Autodesk Inventor part; units mm, degrees
ref_plane "Work Plane1" through (12.7, 0, 0) normal (1, 0, 0) x (0, 1, 0)
ref_plane "Work Plane2" through (0, 12.7, 0) normal (0, 1, 0) x (-1, 0, 0)
ref_plane "Work Plane3" through (0, 0, -12.7) normal (0, 0, 1) x (1, 0, 0)
sketch "Sketch1" plane through (0, 0, 0) normal (0, 1, 0) x (-1, 0, 0)
  line L0 (0, 0) -> (-25.4, 0)
  line L1 (-25.4, 0) -> (-25.4, -25.4)
  line L2 (-25.4, -25.4) -> (0, -25.4)
  line L3 (0, -25.4) -> (0, 0)
  dimension "d0" = 25.4
  dimension "d1" = 25.4
extrude "Extrusion1" add sketch "Sketch1" along normal blind 25.4
sketch "Sketch3" plane through (25.4, 0, 0) normal (1, 0, 0) x (0, 0, -1)
  line L0 (0, 25.4) -> (8.4582, 25.4)
  line L1 (8.4582, 25.4) -> (8.4582, 16.9418)
  line L2 (8.4582, 16.9418) -> (0, 16.9418)
  line L3 (0, 16.9418) -> (0, 25.4)
  line L4 (0, 0) -> (8.4582, 0)
  line L5 (8.4582, 0) -> (8.4582, 8.4582)
  line L6 (8.4582, 8.4582) -> (0, 8.4582)
  line L7 (0, 8.4582) -> (0, 0)
  line L8 (0, 0) -> (25.4, 0)
  line L9 (25.4, 0) -> (16.9418, 0)
  line L10 (16.9418, 0) -> (16.9418, 8.4582)
  line L11 (16.9418, 8.4582) -> (25.4, 8.4582)
  line L12 (25.4, 8.4582) -> (25.4, 0)
  line L13 (0, 25.4) -> (25.4, 25.4)
  line L14 (25.4, 25.4) -> (16.9418, 25.4)
  line L15 (16.9418, 25.4) -> (16.9418, 16.9418)
  line L16 (16.9418, 16.9418) -> (25.4, 16.9418)
  line L17 (25.4, 16.9418) -> (25.4, 25.4)
  line L18 (8.4582, 25.4) -> (16.9418, 25.4)
  line L19 (16.9418, 25.4) -> (16.9418, 0)
  line L20 (16.9418, 0) -> (8.4582, 0)
  line L21 (8.4582, 0) -> (8.4582, 25.4)
  line L22 (0, 16.9418) -> (25.4, 16.9418)
  line L23 (25.4, 16.9418) -> (25.4, 8.4582)
  line L24 (25.4, 8.4582) -> (0, 8.4582)
  line L25 (0, 8.4582) -> (0, 16.9418)
  dimension "d4" = 8.4582
  dimension "d5" = 8.4582
  dimension "d6" = 8.4582
  dimension "d7" = 8.4582
  dimension "d8" = 8.4582
  dimension "d9" = 8.4582
  dimension "d10" = 8.4582
  dimension "d11" = 8.4582
extrude "Extrusion2" cut sketch "Sketch3" against normal blind 2.54 contours L13 L15 L22 L1 | L2 L21 L6 L25 | L22 L19 L24 L21 | L24 L10 L8 L5 | L16 L23 L11 L19
sketch "Sketch5" plane through (25.4, 0, -25.4) normal (0, 0, -1) x (-1, 0, 0)
  line L0 (25.4, 0) -> (25.4, 25.4)
  line L1 (25.4, 0) -> (16.9418, 0)
  line L2 (16.9418, 0) -> (16.9418, 8.4582)
  line L3 (16.9418, 8.4582) -> (25.4, 8.4582)
  line L4 (25.4, 8.4582) -> (25.4, 0)
  line L5 (0, 0) -> (8.4582, 0)
  line L6 (8.4582, 0) -> (8.4582, 8.4582)
  line L7 (8.4582, 8.4582) -> (0, 8.4582)
  line L8 (0, 8.4582) -> (0, 0)
  line L9 (2.54, 25.4) -> (0, 25.4)
  line L10 (0, 25.4) -> (8.4582, 25.4)
  line L11 (8.4582, 25.4) -> (8.4582, 16.9418)
  line L12 (8.4582, 16.9418) -> (0, 16.9418)
  line L13 (0, 16.9418) -> (0, 25.4)
  line L14 (0, 25.4) -> (25.4, 25.4)
  line L15 (25.4, 25.4) -> (16.9418, 25.4)
  line L16 (16.9418, 25.4) -> (16.9418, 16.9418)
  line L17 (16.9418, 16.9418) -> (25.4, 16.9418)
  line L18 (25.4, 16.9418) -> (25.4, 25.4)
  line L19 (0, 8.4582) -> (2.54, 8.4582)
  line L20 (0, 8.4582) -> (25.4, 8.4582)
  line L21 (25.4, 8.4582) -> (25.4, 16.9418)
  line L22 (25.4, 16.9418) -> (0, 16.9418)
  line L23 (0, 16.9418) -> (0, 8.4582)
  line L24 (8.4582, 25.4) -> (16.9418, 25.4)
  line L25 (16.9418, 25.4) -> (16.9418, 0)
  line L26 (16.9418, 0) -> (8.4582, 0)
  line L27 (8.4582, 0) -> (8.4582, 25.4)
  dimension "d14" = 8.4582
  dimension "d15" = 8.4582
  dimension "d16" = 8.4582
  dimension "d17" = 8.4582
  dimension "d18" = 8.4582
  dimension "d19" = 8.4582
  dimension "d20" = 8.4582
  dimension "d21" = 8.4582
extrude "Extrusion3" cut sketch "Sketch5" against normal blind 2.54 contours L3 L25 L17 L0 | L26 L6 L20 L2 | L20 L27 L22 L25 | L22 L11 L14 L16 | L7 L23 L12 L27
sketch "Sketch7" plane through (0, 0, 0) normal (0, -1, 0) x (1, 0, 0)
  line L0 (25.4, -16.9418) -> (25.4, -25.4)
  line L1 (25.4, -25.4) -> (16.9418, -25.4)
  line L2 (16.9418, -25.4) -> (16.9418, -16.9418)
  line L3 (16.9418, -16.9418) -> (25.4, -16.9418)
  line L4 (25.4, -16.9418) -> (25.4, -25.4)
  line L5 (8.4582, -25.4) -> (0, -25.4)
  line L6 (0, -25.4) -> (8.4582, -25.4)
  line L7 (8.4582, -25.4) -> (8.4582, -16.9418)
  line L8 (8.4582, -16.9418) -> (0, -16.9418)
  line L9 (0, -16.9418) -> (0, -25.4)
  line L10 (25.4, -8.4582) -> (25.4, 0)
  line L11 (25.4, 0) -> (16.9418, 0)
  line L12 (16.9418, 0) -> (16.9418, -8.4582)
  line L13 (16.9418, -8.4582) -> (25.4, -8.4582)
  line L14 (25.4, -8.4582) -> (25.4, 0)
  line L15 (0, 0) -> (25.4, 0)
  line L16 (0, 0) -> (8.4582, 0)
  line L17 (8.4582, 0) -> (8.4582, -8.4582)
  line L18 (8.4582, -8.4582) -> (0, -8.4582)
  line L19 (0, -8.4582) -> (0, 0)
  line L20 (16.9418, -25.4) -> (8.4582, -25.4)
  line L21 (8.4582, -25.4) -> (8.4582, 0)
  line L22 (8.4582, 0) -> (16.9418, 0)
  line L23 (16.9418, 0) -> (16.9418, -25.4)
  line L24 (0, -16.9418) -> (25.4, -16.9418)
  line L25 (25.4, -16.9418) -> (25.4, -8.4582)
  line L26 (25.4, -8.4582) -> (0, -8.4582)
  line L27 (0, -8.4582) -> (0, -16.9418)
  dimension "d32" = 8.4582
  dimension "d33" = 8.4582
  dimension "d34" = 8.4582
  dimension "d35" = 8.4582
  dimension "d36" = 8.4582
  dimension "d37" = 8.4582
  dimension "d38" = 8.4582
  dimension "d39" = 8.4582
extrude "Extrusion4" cut sketch "Sketch7" against normal blind 2.54 contours L3 L23 L13 L25 | L24 L21 L26 L23 | L2 L20 L7 L24 | L26 L17 L15 L12 | L8 L27 L18 L21
ref_plane "Work Plane1" through (12.7, 0, 0) normal (1, 0, 0) x (0, 1, 0)
ref_plane "Work Plane2" through (0, 12.7, 0) normal (0, 1, 0) x (-1, 0, 0)
ref_plane "Work Plane3" through (0, 0, -12.7) normal (0, 0, 1) x (1, 0, 0)
mirror "Mirror1" about plane through (12.7, 0, 0) normal (1, 0, 0) of "Extrusion2"
mirror "Mirror2" about plane through (0, 0, -12.7) normal (0, 0, 1) of "Extrusion3"
mirror "Mirror3" about plane through (0, 12.7, 0) normal (0, 1, 0) of "Extrusion4"
ref_plane "Work Plane4" through (0, 12.7, 0) normal (0, 1, 0) x (-1, 0, 0)
properties part number "Portal"
Geometry check sheet. Reference: the model listing, model coordinates, mm. A direction names the side the tool comes from. Coordinates: 2 decimals unless noted, no trailing zeros. Order: outer loops, then holes, each group sorted by start corner. A loop starts at its lowest first (then second) coordinate and runs counter-clockwise, first axis right, second up. Notation, with made-up numbers: (86.25, 8) - (111.25, 8) arc R20 ccw to (111.25, 35) - close; hole circle Ø7 at (6, -1.75). An arc over 180 degrees is marked (long way). Answer in a Markdown table with one row per item. Add a question column.
1) Set-up check for faces 4 (the flat face through (22, 16.942, -2)), 5 (the flat face through (2, 22, -8.458)), 6 (the flat face through (2, 3, -16.942)), 7 (the flat face through (22.1, 16.942, -23.1)): record each of +Z, -Z, +X, -X, +Y, -Y from which the full face is reachable in a straight line by a thin tool's end or side.
2) Gauge pin test, flat ends, axial feed: P1, Ø4, axis at y = 10.5, z = -16.5, coming from the +X side; P2, Ø4, axis at x = 14, z = -5.5, coming from the +Y side; P3, Ø1.5, axis at x = 14, y = 6.5, coming from the -Z side. Record the tip position at first contact, or that the pin passes through.
3) Cross-section at A-A, the plane x = 20.75. Record the cut outline in (y, z).
4) Cross-section at D-D, the plane z = -16.25. Record the cut outline in (x, y).
5) Cross-section at C-C, the plane y = 9.5. Record the cut outline in (x, z), then the cut area to 3 significant figures.
6) Material ranges on line 1 along X through (y, z) = (3.75, -2); line 2 along Y through (x, z) = (9, -20.5); line 3 along Z through (x, y) = (8.75, 7.5), recorded low to high. Write a range as [from, to].
7) Release check for a two-part mould opening along Z. For faces 1 (the flat face through (13, 2.54, -13)), 2 (the flat face through (21, 0, -4)), 3 (the flat face through (21, 21, 0)) record: +Z half, -Z half, draft (parallel to the pull), parting line (faces both ways), or undercut.
8) Cross-section at B-B, the plane z = -19.25. Record the cut outline in (x, y), then the cut area to 3 significant figures.
Check result:
| question | item | result |
|---|---|---|
| 1 | face 4 | +Z, +X |
| 1 | face 5 | -X, +Y |
| 1 | face 6 | -X, -Y |
| 1 | face 7 | -Z, +X |
| 2 | P1 | stops at x = 22.86 |
| 2 | P2 | stops at y = 22.86 |
| 2 | P3 | stops at z = -22.86 |
| 3 | outline | (0, -25.4) - (8.46, -25.4) - (8.46, -22.86) - (16.94, -22.86) - (16.94, -25.4) - (25.4, -25.4) - (25.4, -16.94) - (22.86, -16.94) - (22.86, -8.46) - (25.4, -8.46) - (25.4, 0) - (16.94, 0) - (16.94, -2.54) - (8.46, -2.54) - (8.46, 0) - (0, 0) - (0, -8.46) - (2.54, -8.46) - (2.54, -16.94) - (0, -16.94) - close |
| 4 | outline | (2.54, 2.54) - (22.86, 2.54) - (22.86, 22.86) - (2.54, 22.86) - close |
| 5 | outline | (2.54, -22.86) - (22.86, -22.86) - (22.86, -2.54) - (2.54, -2.54) - close |
| 5 | area | 413 mm² |
| 6 | line 1 | x = [0, 8.46], [16.94, 25.4] |
| 6 | line 2 | y = [2.54, 22.86] |
| 6 | line 3 | z = [-22.86, -2.54] |
| 7 | face 1 | undercut |
| 7 | face 2 | draft |
| 7 | face 3 | +Z half |
| 8 | outline | (0, 0) - (8.46, 0) - (8.46, 2.54) - (16.94, 2.54) - (16.94, 0) - (25.4, 0) - (25.4, 8.46) - (22.86, 8.46) - (22.86, 16.94) - (25.4, 16.94) - (25.4, 25.4) - (16.94, 25.4) - (16.94, 22.86) - (8.46, 22.86) - (8.46, 25.4) - (0, 25.4) - (0, 16.94) - (2.54, 16.94) - (2.54, 8.46) - (0, 8.46) - close |
| 8 | area | 559 mm² |
